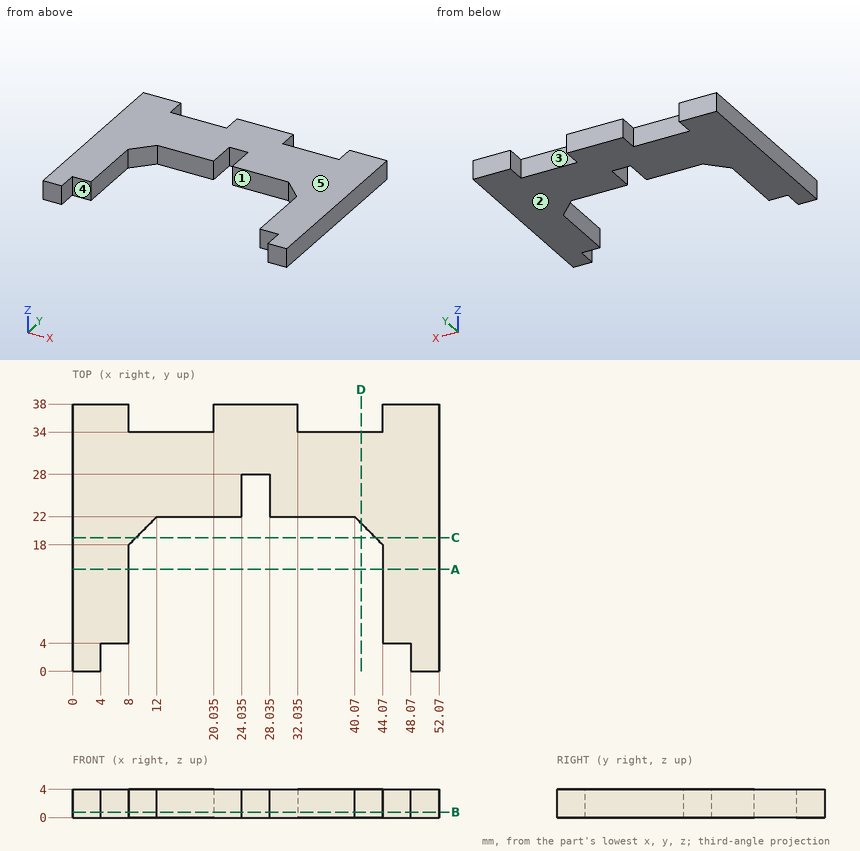
Design review of the part shown in the three views and the two pictorial views. Dimensions are in mm from the part's minimum x, y and z. A direction names the side the tool comes from. Give positions to 0.01 mm unless a question says otherwise; leave off trailing zeros. Loops run counter-clockwise (first coordinate to the right, second up) from the corner with the lowest first, then second, coordinate; pieces in that order, holes last. Notation, with made-up numbers: M 62,38.25 L 114,38.25 A30 cw 114,62.25 Z; hole C 72,88 d5. An arc over 180 degrees is marked long. Write item = value, one per line.
Q1. Draft analysis for pull direction X (two halves, no side actions). For the marked faces 4 and 5, state which applies: +X half, -X half, draft (parallel to the pull), parting line (faces both ways), or undercut.
Output values:
face_4 = undercut
face_5 = draft
Q2. We need section A-A (y = 14.5). Give the boundary of the cut face in (x, z), plus the area to 3 significant figures.
Output values:
outline = M 0,0 L 8,0 L 8,4 L 0,4 Z; M 44.07,0 L 52.07,0 L 52.07,4 L 44.07,4 Z
area = 64.0 mm^2
Q3. We need section C-C (y = 19). Give the boundary of the cut face in (x, z).
Output values:
outline = M 0,0 L 9,0 L 9,4 L 0,4 Z; M 43.07,0 L 52.07,0 L 52.07,4 L 43.07,4 Z
Q4. For the marked faces 1, 2 and 3, list the 3-axis set-ups (+Z, -Z, +X, -X, +Y, -Y) from which the entire face can be reached by the end or side of a thin tool; tool diameter is ignored.
Output values:
face_1 = +Z, -Z, -Y
face_2 = -Z, +X, -X, +Y, -Y
face_3 = +Z, -Z, +Y
Q5. We need section D-D (x = 41). Give the boundary of the cut face in (y, z), plus the area to 3 significant figures.
Output values:
outline = M 21.07,0 L 34,0 L 34,4 L 21.07,4 Z
area = 51.7 mm^2
Q6. To check wall thickness, follow line 1 (X direction, y = 35.5, z = 2.1) (3 decimals); line 2 (X direction, y = 13, z = 2.2); line 3 (X direction, y = 24, z = 1.6) (3 decimals). State the ranges of each line that lie inside material, in increasing order. Write a range as [from, to].
Output values:
line_1 = [0, 8], [20.035, 32.035], [44.07, 52.07]
line_2 = [0, 8], [44.07, 52.07]
line_3 = [0, 24.035], [28.035, 52.07]
Q7. Insertion check: pin 1 (1.2 mm diameter, centred on x = 46, z = 2, fed in from -Y); pin 2 (1 mm diameter, centred on x = 41, z = 1.5, fed in from +Y); pin 3 (2 mm diameter, centred on x = 17.5, z = 2, fed in from -Y); pin 4 (3 mm diameter, centred on x = 10, y = 6, fed in from +Z). Each pin has a flat end and moves straight along its axis. Give the tip position at first contact, or say it passes through.
Output values:
pin_1 = 4
pin_2 = 34
pin_3 = 22
pin_4 = through
Q8. We need section B-B (z = 0.8). Give the boundary of the cut face in (x, y) (3 decimals), plus the area to 3 significant figures.
Output values:
outline = M 0,0 L 4,0 L 4,4 L 8,4 L 8,18 L 12,22 L 24.035,22 L 24.035,28 L 28.035,28 L 28.035,22 L 40.07,22 L 44.07,18 L 44.07,4 L 48.07,4 L 48.07,0 L 52.07,0 L 52.07,38 L 44.07,38 L 44.07,34 L 32.035,34 L 32.035,38 L 20.035,38 L 20.035,34 L 8,34 L 8,38 L 0,38 Z
area = 1,050 mm^2
